```python
from build123d import *

# Parameters (mm, degrees)
EXTRUDE_1_DEPTH = 12
FILLET_1_R      = 2


with BuildPart() as part:
    # Эскиз1 → Бобышка-Вытянуть1 (new body)
    with BuildSketch(Plane.XY):
        with BuildLine():
            Line((0, 0), (5, 0))
            Line((5, 0), (5, 20))
            Line((5, 20), (17, 20))
            Line((17, 20), (17, 0))
            Line((17, 0), (22, 0))
            Line((22, 0), (22, 18.757359313))
            ThreePointArc((22, 18.757359313), (22.228361402, 19.90540961), (22.878679656, 20.878679656))
            Line((22.878679656, 20.878679656), (34.624442368, 32.624442368))
            ThreePointArc((34.624442368, 32.624442368), (35.503122025, 34.745762712), (34.624442368, 36.867083055))
            Line((34.624442368, 36.867083055), (24.799286445, 46.692238978))
            ThreePointArc((24.799286445, 46.692238978), (22.677966102, 47.570918635), (20.556645758, 46.692238978))
            Line((20.556645758, 46.692238978), (0, 26.13559322))
            Line((0, 26.13559322), (0, 0))
        make_face()
    extrude(amount=EXTRUDE_1_DEPTH)

    # Скругление1
    fillet_1_edges = [part.edges().sort_by_distance(p)[0] for p in [
        (0, 26.13559322, 6),
        (22, 0, 6),
        (17, 0, 6),
        (17, 20, 6),
        (5, 20, 6),
        (5, 0, 6),
        (0, 0, 6),
    ]]
    fillet(fillet_1_edges, radius=FILLET_1_R)


solid = part.part
```
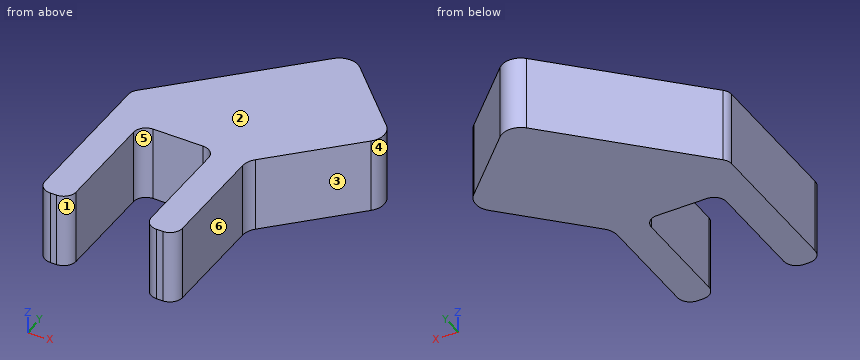
Could you check a few things on this model? Use its own coordinates, in mm. Face numbers are marked on the shaded views. A direction names the side the tool comes from. Coordinates: 2 decimals unless noted, no trailing zeros. Write each loop counter-clockwise with the first axis right and the second up, starting at its lowest first coordinate (ties: lowest second). Pieces come first, ordered by that corner, then holes. Notation, with made-up numbers: (42, 27) - (77, 27) arc R14 cw to (77, 46) - close; hole circle Ø9 at (33, -18.75). An arc over 180 degrees is marked (long way). Use a Markdown table: item, result.
Q1. Which directions (+Z, -Z, +X, -X, +Y, -Y) give clear straight access to the entire face, cutting with the end or side of a thin tool? Please do the marked faces 4, 5 and 6.
Geometry check:
| item | result |
|---|---|
| face 4 | +Z, -Z, +X |
| face 5 | +Z, -Z, -Y |
| face 6 | +Z, -Z, +X, -Y |
Q2. Please list where these lines run through material, in increasing order: L1, parallel to X at y = 14, z = 1.75; L2, parallel to X at y = 37.5, z = 1.5; L3, parallel to Y at x = 14.5, z = 11.75.
Geometry check:
| item | result |
|---|---|
| L1 | x = 0 to 5, 17 to 22 |
| L2 | x = 11.36 to 33.99 |
| L3 | y = 20 to 40.64 |
Q3. I'm going to push flat-ended pins straight in: pin 1 Ø3.5 at (y, z) = (13.5, 4) entering from +X; pin 2 Ø1 at (x, z) = (9, 6.5) entering from +Y; pin 3 Ø8 at (x, y) = (26.5, 18) entering from +Z; pin 4 Ø1.5 at (x, z) = (25.5, 9) entering from -Y. Where does each tip first touch, or does it pass through?
Geometry check:
| item | result |
|---|---|
| pin 1 | stops at x = 22 |
| pin 2 | stops at y = 35.64 |
| pin 3 | passes through |
| pin 4 | stops at y = 22.75 |
Q4. Thinking about a two-plate mould opening in X: for the marked faces 1, 2 and 3, which applies, +X half, -X half, draft (parallel to the pull), parting line (faces both ways), or undercut?
Geometry check:
| item | result |
|---|---|
| face 1 | undercut |
| face 2 | draft |
| face 3 | +X half |
Q5. Imagine slicing it at D-D (x = 6). List the corners of the cut face in (y, z) for me, and give its area (3 significant figures).
Geometry check:
| item | result |
|---|---|
| outline | (19.73, 0) - (32.14, 0) - (32.14, 12) - (19.73, 12) - close |
| area | 149 mm2 |
Q6. Imagine slicing it at C-C (y = 21.5). List the corners of the cut face in (x, z) for me, and give its area (3 significant figures).
Geometry check:
| item | result |
|---|---|
| outline | (0, 0) - (23.5, 0) - (23.5, 12) - (0, 12) - close |
| area | 282 mm2 |
Q7. Imagine slicing it at A-A (y = 16). List the corners of the cut face in (x, z) for me, and give its area (3 significant figures).
Geometry check:
| item | result |
|---|---|
| outline | (0, 0) - (5, 0) - (5, 12) - (0, 12) - close; (17, 0) - (22, 0) - (22, 12) - (17, 12) - close |
| area | 120 mm2 |
Q8. Imagine slicing it at B-B (z = 1.25). List the corners of the cut face in (x, y) for me, and give its area (3 significant figures).
Geometry check:
| item | result |
|---|---|
| outline | (0, 2) arc R2 ccw to (2, 0) - (3, 0) arc R2 ccw to (5, 2) - (5, 18) arc R2 cw to (7, 20) - (15, 20) arc R2 cw to (17, 18) - (17, 2) arc R2 ccw to (19, 0) - (20, 0) arc R2 ccw to (22, 2) - (22, 18.76) arc R3 cw to (22.88, 20.88) - (34.62, 32.62) arc R3 ccw to (34.62, 36.87) - (24.8, 46.69) arc R3 ccw to (20.56, 46.69) - (0.59, 26.72) arc R2 ccw to (0, 25.31) - close |
| area | 788 mm2 |
